Autodesk Inventor part; units mm, degrees
ref_plane "YZ Plane" through (0, 0, 0) normal (1, 0, 0) x (0, 1, 0)
ref_plane "XZ Plane" through (0, 0, 0) normal (0, 1, 0) x (-1, 0, 0)
ref_plane "XY Plane" through (0, 0, 0) normal (0, 0, 1) x (1, 0, 0)
sketch "Esquisse1" plane through (0, 0, 0) normal (0, 1, 0) x (-1, 0, 0)
  circle A0 centre (0, 0) radius 7.25
  dimension "d0" = 14.5
extrude "Extrusion1" add sketch "Esquisse1" along normal blind 3
sketch "Esquisse2" plane through (0, 3, 0) normal (0, 1, 0) x (1, 0, 0)
  circle A0 centre (0, 0) radius 6
  dimension "d3" = 12
extrude "Extrusion2" add sketch "Esquisse2" along normal blind 16
sketch "Esquisse3" plane through (0, 19, 0) normal (0, 1, 0) x (1, 0, 0)
  circle A0 centre (0, 0) radius 5.5
  dimension "d6" = 11
extrude "Extrusion3" add sketch "Esquisse3" along normal blind 5
thread "Filetage1"
sketch "Esquisse4" plane through (0, 24, 0) normal (0, 1, 0) x (1, 0, 0)
  line L0 (-7.5, 3) -> (-5.5, 3)
  line L1 (-5.5, 3) -> (-5.5, -3)
  line L2 (-5.5, -3) -> (-7.5, -3)
  line L3 (-7.5, -3) -> (-7.5, 3)
  line L4 (7.5, 3) -> (5.5, 3)
  line L5 (5.5, 3) -> (5.5, -3)
  line L6 (5.5, -3) -> (7.5, -3)
  line L7 (7.5, -3) -> (7.5, 3)
  circle A0 centre (0, 0) radius 5.5
  circle A1 centre (0, 0) radius 5.5
  point P0 (-5.5, 0)
  point P1 (5.5, 0)
  dimension "d11" = 2
  dimension "d12" = 11
  dimension "d13" = 5.5
  dimension "d14" = 5.5
  dimension "d15" = 11
  dimension "d16" = 2
  dimension "d17" = 6
  dimension "d18" = 3
extrude "Extrusion4" cut sketch "Esquisse4" against normal blind 21 contours L5 L4 L7 L6 | L0 L1 L2 L3
sketch "Esquisse5" plane through (0, 24, 0) normal (0, 1, 0) x (1, 0, 0)
  line L0 (-0.5, 3) -> (0.5, 3)
  line L1 (0.5, 3) -> (0.5, -3)
  line L2 (0.5, -3) -> (-0.5, -3)
  line L3 (-0.5, -3) -> (-0.5, 3)
  point P0 (0, 0)
  dimension "d21" = 1
  dimension "d22" = 0.5
  dimension "d23" = 6
  dimension "d24" = 3
extrude "Extrusion5" add sketch "Esquisse5" along normal blind 10
sketch "Esquisse6" plane through (0, 0, 0) normal (0, -1, 0) x (1, 0, 0)
  circle A0 centre (0, 0) radius 5
  circle A1 centre (0, 0) radius 3
  circle A2 centre (0, 0) radius 2.5
  dimension "d27" = 10
  dimension "d28" = 6
  dimension "d29" = 5
extrude "Extrusion6" cut sketch "Esquisse6" against normal blind 10
chamfer "Chanfrein1" distance 0.5 angle 45 6 edges at (7.25, 0, 0) (-5.5, 24, 0) (0, 34, -3) (0, 34, 3) (0.5, 34, 0) (-0.5, 34, 0)
sketch "Esquisse7" plane through (0.5, 24, 3) normal (1, 0, 0) x (0, 0, -1)
  circle A0 centre (3, 6) radius 0.75
  line L0 (-2, 0) -> (8, 0)
  point P0 (3, -24)
  dimension "d35" = 1.5
  dimension "d36" = 6
extrude "Extrusion7" cut sketch "Esquisse7" against normal blind 10
equation "\"d15\" = d12"
equation "\"d16\" = d11"
equation "\"d18\" = 0.5 * d17"
properties part number "Prise banane" material "Plastique ABS"
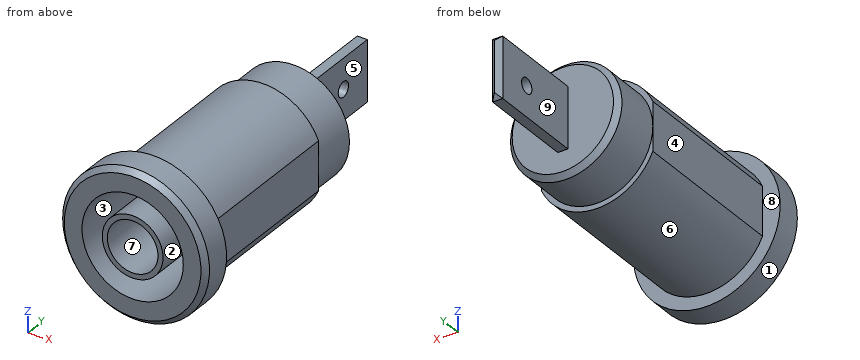
Input: part model. Units: mm. Frame: model coordinates. Face numbers are marked on the shaded views. A direction names the side the tool comes from. Coordinates: 2 decimals unless noted, no trailing zeros. Order: outer loops, then holes, each group sorted by start corner. A loop starts at its lowest first (then second) coordinate and runs counter-clockwise, first axis right, second up. Notation, with made-up numbers: M 54,23.25 L 93,23.25 A8 ccw 93,27.25 Z; hole C 59,47.25 d5. An arc over 180 degrees is marked long. Write item = value, one per line. Start each with the question number.
(1) Section C-C on y = 2. Output: boundary loops of the cut face in (x, z), and give its area (3 significant figures).
(2) Section B-B on y = 30. Output: boundary loops of the cut face in (x, z).
(3) Line query: line 1 along Z through (x, y) = (0, 8); line 2 along X through (y, z) = (5, -1); line 3 along X through (y, z) = (32.5, 2.75). Output: solid intervals per line, ascending. Write a range as [from, to].
(4) First-contact query: P1, Ø6.5, axis at x = -0.5, z = 3, coming from the +Y side; P2, Ø0.5, axis at x = 0, y = 28.5, coming from the -Z side; P3, Ø1, axis at x = -0.5, y = 10, coming from the -Z side; P4, Ø4, axis at x = 0, z = 0, coming from the -Y side. Flat tips, straight axial feed; report the tip coordinate or a pass-through.
(5) Section A-A on y = 7.5. Output: boundary loops of the cut face in (x, z).
(6) Section D-D on y = 14. Output: boundary loops of the cut face in (x, z).
(7) Pull-direction query (Z, two-part tool) for the marked faces 1, 2, 3 and 4; classes: released by +Z, released by -Z, zero draft, split by the parting line, or undercut.
(8) Reachability of the marked faces 5, 6, 7, 8 and 9 from +Z, -Z, +X, -X, +Y, -Y: full face, straight path, thin tool, end or side. Return the list, or none.
Result set:
q1.outline = C 0,0 d14.5; C 0,0 d6; hole C 0,0 d10; hole C 0,0 d5
q1.area = 95.2 mm²
q2.outline = M -0.5,-3 L 0.5,-3 L 0.5,-0.75 L -0.5,-0.75 Z; M -0.5,0.75 L 0.5,0.75 L 0.5,3 L -0.5,3 Z
q3.line_1 = [-6, -5], [-3, -2.5], [2.5, 3], [5, 6]
q3.line_2 = [-5.5, -4.9], [-2.83, -2.29], [2.29, 2.83], [4.9, 5.5]
q3.line_3 = [-0.5, 0.5]
q4.P1 = 34
q4.P2 = -3
q4.P3 = -6
q4.P4 = 10
q5.outline = M -5.5,-2.4 A6 ccw 5.5,-2.4 L 5.5,2.4 A6 ccw -5.5,2.4 Z; C 0,0 d6; hole C 0,0 d10; hole C 0,0 d5
q6.outline = M -5.5,-2.4 A6 ccw 5.5,-2.4 L 5.5,2.4 A6 ccw -5.5,2.4 Z
q7.face_1 = split by the parting line
q7.face_2 = undercut
q7.face_3 = undercut
q7.face_4 = zero draft
q8.face_5 = +Z, -Z, +X, +Y
q8.face_6 = -Z, +Y
q8.face_7 = -Y
q8.face_8 = +Y
q8.face_9 = +Z, -Z, -X, +Y
